Source: three-view drawing plus pictorial views. Frame: mm from the lowest corner of the part. A direction names the side the tool comes from. Give positions to 0.01 mm unless a question says otherwise; leave off trailing zeros. Write each loop counter-clockwise with the first axis right and the second up, starting at its lowest first coordinate (ties: lowest second). Pieces come first, ordered by that corner, then holes. Notation, with made-up numbers: M 56,63 L 68,63 A24 cw 68,75 Z; hole C -30,38.5 d7. An arc over 180 degrees is marked long. One line per question, with ' | ' between items.
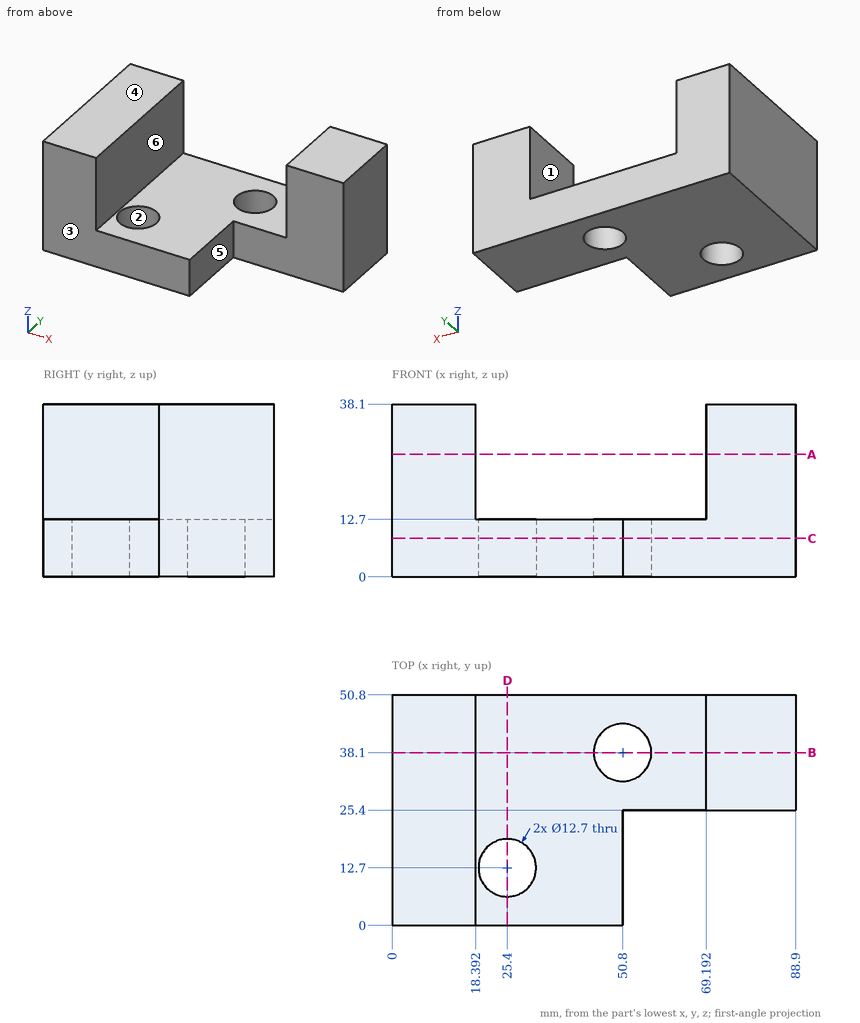
(1) Cut plane B-B, the plane y = 38.1. Return loops of the section in (x, z), then the cut area to 3 significant figures.
Working result:
outline: M 0,0 L 44.45,0 L 44.45,12.7 L 18.39,12.7 L 18.39,38.1 L 0,38.1 Z; M 57.15,0 L 88.9,0 L 88.9,38.1 L 69.19,38.1 L 69.19,12.7 L 57.15,12.7 Z | area: 1,940 mm^2
(2) Cut plane A-A, the plane z = 27. Return loops of the section in (x, y), then the cut area to 3 significant figures.
Working result:
outline: M 0,0 L 18.39,0 L 18.39,50.8 L 0,50.8 Z; M 69.19,25.4 L 88.9,25.4 L 88.9,50.8 L 69.19,50.8 Z | area: 1,430 mm^2
(3) Draft query along Y for the marked faces 1, 2 and 3. Return one class per face: released by +Y, released by -Y, zero draft, split by the parting line, or undercut.
Working result:
face 1: zero draft | face 2: undercut | face 3: released by -Y
(4) Material intervals for L1, parallel to Y at x = 25, z = 4; L2, parallel to X at y = 36, z = 25; L3, parallel to Z at x = 54, y = 29, sorted ascending. Write a range as [from, to].
Working result:
L1: y = [0, 6.36], [19.04, 50.8] | L2: x = [0, 18.39], [69.19, 88.9] | L3: z = [0, 12.7]
(5) Set-up query: the marked faces 4, 5 and 6. Return all of +Z, -Z, +X, -X, +Y, -Y with unobstructed straight access to the full face (end or side cutting, diameter ignored); none if empty.
Working result:
face 4: +Z, +X, -X, +Y, -Y | face 5: +Z, -Z, +X, -Y | face 6: +Z, +Y, -Y
(6) First-contact query: P1, Ø8, axis at x = 59, y = 25, coming from the +Z side; P2, Ø1.5, axis at x = 42, y = 21, coming from the -Z side; P3, Ø11.5, axis at x = 66.5, z = 14, coming from the -Y side; P4, Ø10, axis at x = 63.5, y = 16, coming from the +Z side. Flat tips, straight axial feed; report the tip coordinate or a pass-through.
Working result:
P1: stops at z = 12.7 | P2: stops at z = 0 | P3: stops at y = 25.4 | P4: passes through
(7) Cut plane C-C, the plane z = 8.5. Return loops of the section in (x, y), then the cut area to 4 significant figures.
Working result:
outline: M 0,0 L 50.8,0 L 50.8,25.4 L 88.9,25.4 L 88.9,50.8 L 0,50.8 Z; hole C 25.4,12.7 d12.7; hole C 50.8,38.1 d12.7 | area: 3,295 mm^2
(8) Cut plane D-D, the plane x = 25.4. Return loops of the section in (y, z).
Working result:
outline: M 0,0 L 6.35,0 L 6.35,12.7 L 0,12.7 Z; M 19.05,0 L 50.8,0 L 50.8,12.7 L 19.05,12.7 Z
